from build123d import *

# Parameters (mm, degrees)
F0_W     = 70.7883353009
F0_H     = 70.6329355565
F1_DEPTH = 6
F2_R     = 49.1
F3_DEPTH = 5.2
F4_R     = 29.1804773136
F5_DEPTH = 25


with BuildPart() as f1:
    # F0 (on Front) → F1 (new body)
    with BuildSketch(Plane.XZ):
        with BuildLine():
            ThreePointArc((35.3941676505, -35.3164677782), (46.204482372, -19.1087887826), (50, 0))
            ThreePointArc((50, 0), (46.5418074661, 18.2718405693), (36.6455936884, 34.0161794331))
            ThreePointArc((36.6455936884, 34.0161794331), (36.0257476104, 34.6719700784), (35.3941676505, 35.3164677782))
            Line((35.3941676505, 35.3164677782), (35.3941676505, -35.3164677782))
        make_face()
        with BuildLine():
            ThreePointArc((35.3941676505, 35.3164677782), (36.0257476104, 34.6719700784), (36.6455936884, 34.0161794331))
            Line((36.6455936884, 34.0161794331), (70.0867437781, 71.187263365))
            Line((70.0867437781, 71.187263365), (68.7485847566, 72.3911447683))
            Line((68.7485847566, 72.3911447683), (35.3941676505, 35.3164677782))
        make_face()
        with BuildLine():
            Line((70.9903525089, -70.3661009157), (35.3941676505, -35.3164677782))
            ThreePointArc((35.3941676505, -35.3164677782), (34.7525403407, -35.9480310986), (34.0996454535, -36.5679392357))
            Line((34.0996454535, -36.5679392357), (69.7274450602, -71.6487017016))
            Line((69.7274450602, -71.6487017016), (70.9903525089, -70.3661009157))
        make_face()
        with BuildLine():
            ThreePointArc((34.0996454535, -36.5679392357), (34.7525403407, -35.9480310986), (35.3941676505, -35.3164677782))
            Line((35.3941676505, -35.3164677782), (-35.3941676505, -35.3164677782))
            ThreePointArc((-35.3941676505, -35.3164677782), (-34.7527012082, -35.9478755803), (-34.0999727359, -36.5676340418))
            ThreePointArc((-34.0999727359, -36.5676340418), (-0.0002237505, -49.9999999995), (34.0996454535, -36.5679392357))
        make_face()
        Rectangle(F0_W, F0_H)
        with BuildLine():
            Line((-35.3941676505, 35.3164677782), (35.3941676505, 35.3164677782))
            ThreePointArc((35.3941676505, 35.3164677782), (0, 50), (-35.3941676505, 35.3164677782))
        make_face()
        with BuildLine():
            ThreePointArc((-36.6424362928, 34.0195805754), (-49.9918991162, -0.9000126416), (-35.3941676505, -35.3164677782))
            Line((-35.3941676505, -35.3164677782), (-35.3941676505, 35.3164677782))
            ThreePointArc((-35.3941676505, 35.3164677782), (-36.0241385188, 34.6736419197), (-36.6424362928, 34.0195805754))
        make_face()
        with BuildLine():
            ThreePointArc((-34.0999727359, -36.5676340418), (-34.7527012082, -35.9478755803), (-35.3941676505, -35.3164677782))
            Line((-35.3941676505, -35.3164677782), (-70.5225346289, -70.8973310818))
            Line((-70.5225346289, -70.8973310818), (-69.24162355, -72.161952293))
            Line((-69.24162355, -72.161952293), (-34.0999727359, -36.5676340418))
        make_face()
        with BuildLine():
            ThreePointArc((-36.6424362928, 34.0195805754), (-36.0241385188, 34.6736419197), (-35.3941676505, 35.3164677782))
            Line((-35.3941676505, 35.3164677782), (-71.2271848866, 70.1739048632))
            Line((-71.2271848866, 70.1739048632), (-72.4822921078, 68.8836700538))
            Line((-72.4822921078, 68.8836700538), (-36.6424362928, 34.0195805754))
        make_face()
    extrude(amount=F1_DEPTH)

    # F2 (on Front) → F3 (cut)
    with BuildSketch(Plane.XZ):
        Circle(F2_R)
    extrude(amount=F3_DEPTH, mode=Mode.SUBTRACT)

    # F4 (on Front) → F5 (cut)
    with BuildSketch(Plane.XZ):
        Circle(F4_R)
    extrude(amount=F5_DEPTH, mode=Mode.SUBTRACT)


solid = f1.part
Model file for the job. Use its own axes, mm. A direction names the side the tool comes from. Give positions to 0.01 mm unless a question says otherwise; leave off trailing zeros. Order: outer loops, then holes, each group sorted by start corner. A loop starts at its lowest first (then second) coordinate and runs counter-clockwise, first axis right, second up. Notation, with made-up numbers: (-6.75, 42.5) - (46.25, 42.5) arc R28 ccw to (46.25, 73.5) - close; hole circle Ø5 at (33, -2.75). An arc over 180 degrees is marked (long way). One line per item, written item: value.
Item 1: Slice it at C-C (y = -1.4). List the corners of the cut face in (x, z), then the cut area to 3 significant figures.
Response values:
outline: (-72.48, 68.88) - (-36.64, 34.02) arc R50 ccw to (-35.39, -35.32) - (-70.52, -70.9) - (-69.24, -72.16) - (-34.1, -36.57) arc R50 ccw to (34.1, -36.57) - (69.73, -71.65) - (70.99, -70.37) - (35.39, -35.32) arc R50 ccw to (36.65, 34.02) - (70.09, 71.19) - (68.75, 72.39) - (35.39, 35.32) arc R50 ccw to (-35.39, 35.32) - (-71.23, 70.17) - close; hole circle Ø98.2 at (0, 0)
area: 640 mm2
Item 2: Pin check, flat tips, straight feed: pin 1 Ø1 at (x, y) = (-51.5, -5) entering from -Z; pin 2 Ø2 at (x, y) = (-52, -5) entering from -Z; pin 3 Ø12 at (x, z) = (15, 56) entering from +Y. Stop position of each tip, or through.
Response values:
pin 1: z = -54.7
pin 2: z = -55.71
pin 3: through
Item 3: Wall check: line 1 (Z direction, x = 0, y = -3.5); line 2 (Z direction, x = 0, y = -5.35); line 3 (Z direction, x = -44.5, y = -4.4). Give the ranges that are in metal, low to high.
Response values:
line 1: -50 to -49.1, 49.1 to 50
line 2: -50 to -29.18, 29.18 to 50
line 3: -47.1 to -44.54, -22.8 to -20.75, 20.75 to 22.8, 41.66 to 44.17
Item 4: Tool access for faces 4 (the flat face through (51.7, -3, -53.9)), 5 (the flat face through (52.3, -2.96, 54.11)), 6 (the flat face through (53.441, -2.958, -53.087)), 7 (the flat face through (-54.813, -2.958, 51.696)), 8 (the cylindrical face through (-10.644, -2.564, -47.932)): list every direction of +Z, -Z, +X, -X, +Y, -Y with a clear straight run to the whole face (end or side of a thin tool).
Response values:
face 4: -Z, +Y, -Y
face 5: +Z, +Y, -Y
face 6: +X, +Y, -Y
face 7: -X, +Y, -Y
face 8: +Y
Item 5: Slice it at B-B (z = 46.5). List the corners of the cut face in (x, y).
Response values:
outline: (-49.47, -6) - (-46.89, -6) - (-46.89, 0) - (-49.47, 0) - close; (-18.38, -6) - (18.38, -6) - (18.38, 0) - (15.77, 0) - (15.77, -5.2) - (-15.77, -5.2) - (-15.77, 0) - (-18.38, 0) - close; (45.46, -6) - (47.88, -6) - (47.88, 0) - (45.46, 0) - close
Item 6: Slice it at D-D (x = 57.5). List the corners of the cut face in (y, z), then the cut area to 3 significant figures.
Response values:
outline: (-6, -59.61) - (0, -59.61) - (0, -57.08) - (-6, -57.08) - close; (-6, 57.2) - (0, 57.2) - (0, 59.89) - (-6, 59.89) - close
area: 31.3 mm2
Item 7: Two-plate mould, pull along Z, no slides. Class faces 1 (the flat face through (-53.06, -2.96, 52.5)), 2 (the flat face through (-52.712, -2.958, -52.858)), 3 (the flat face through (-51.917, -2.958, -54.614)): released by +Z, released by -Z, zero draft, split by the parting line, or undercut.
Response values:
face 1: released by +Z
face 2: undercut
face 3: released by -Z
Item 8: Slice it at A-A (x = 0). List the corners of the cut face in (y, z), then the cut area to 3 significant figures.
Response values:
outline: (-6, -50) - (0, -50) - (0, -49.1) - (-5.2, -49.1) - (-5.2, -29.18) - (-6, -29.18) - close; (-6, 29.18) - (-5.2, 29.18) - (-5.2, 49.1) - (0, 49.1) - (0, 50) - (-6, 50) - close
area: 42.7 mm2
